Build history of the part. All positions in model axes, mm. Coordinates: 2 decimals unless noted, no trailing zeros. Loops run counter-clockwise (first coordinate to the right, second up) from the corner with the lowest first, then second, coordinate; pieces in that order, holes last. Notation, with made-up numbers: (-19, 19.5) -> (26, 19.5) arc R17 cw to (26, 42.5) -> close; hole circle Ø3 at (39.25, 50). An arc over 180 degrees is marked (long way). One line per item, written item: value. Start each with the question number.
Autodesk Inventor part; units mm, degrees
ref_plane "YZ Plane" through (0, 0, 0) normal (1, 0, 0) x (0, 1, 0)
ref_plane "XZ Plane" through (0, 0, 0) normal (0, 1, 0) x (-1, 0, 0)
ref_plane "XY Plane" through (0, 0, 0) normal (0, 0, 1) x (1, 0, 0)
sketch "Sketch1" plane through (0, 0, 0) normal (0, 1, 0) x (-1, 0, 0)
  line L0 (0, 0) -> (127, 0)
  line L1 (127, 0) -> (127, -127)
  line L2 (127, -127) -> (0, -127)
  line L3 (0, -127) -> (0, 0)
  line L4 (123.825, 0) -> (127, 0)
  line L5 (127, 0) -> (127, -33.615)
  line L6 (127, -33.615) -> (123.825, -33.615)
  line L7 (123.825, -33.615) -> (123.825, 0)
  line L8 (123.825, -33.615) -> (70.363, -33.615)
  line L9 (70.363, -33.615) -> (70.363, -36.79)
  line L10 (70.363, -36.79) -> (127, -36.79)
  line L11 (70.363, -36.79) -> (67.188, -36.79)
  line L12 (67.188, -36.79) -> (67.188, 0)
  line L13 (67.188, 0) -> (70.363, 0)
  line L14 (70.363, 0) -> (70.363, -36.79)
  line L15 (69.1283, -45.3517) -> (43.7283, -45.3517)
  line L16 (43.7283, -45.3517) -> (43.7283, -42.1767)
  line L17 (43.7283, -42.1767) -> (69.1283, -42.1767)
  line L18 (69.1283, -42.1767) -> (69.1283, -45.3517)
  line L19 (69.1283, -42.1767) -> (72.3033, -42.1767)
  line L20 (72.3033, -42.1767) -> (72.3033, -84.8107)
  line L21 (72.3033, -84.8107) -> (69.1283, -84.8107)
  line L22 (69.1283, -84.8107) -> (69.1283, -42.1767)
  line L23 (69.1283, -84.8107) -> (12.4863, -84.8107)
  line L24 (12.4863, -84.8107) -> (12.4863, -81.6357)
  line L25 (12.4863, -81.6357) -> (69.1283, -81.6357)
  line L26 (69.1283, -81.6357) -> (69.1283, -84.8107)
  line L27 (12.4863, -81.6357) -> (15.6613, -81.6357)
  line L28 (15.6613, -81.6357) -> (15.6613, -42.1767)
  line L29 (15.6613, -42.1767) -> (12.4863, -42.1767)
  line L30 (12.4863, -42.1767) -> (12.4863, -81.6357)
  line L31 (127, -90.21) -> (67.188, -90.21)
  line L32 (67.188, -90.21) -> (67.188, -93.385)
  line L33 (67.188, -93.385) -> (127, -93.385)
  line L34 (127, -93.385) -> (127, -90.21)
  line L35 (127, -93.385) -> (123.825, -93.385)
  line L36 (123.825, -93.385) -> (123.825, -127)
  line L37 (123.825, -127) -> (127, -127)
  line L38 (127, -127) -> (127, -93.385)
  line L39 (25.4, 0) -> (6.35, 0)
  line L40 (25.4, -127) -> (6.35, -127)
  line L41 (67.188, -90.21) -> (70.363, -90.21)
  line L42 (70.363, -90.21) -> (70.363, -127)
  line L43 (70.363, -127) -> (67.188, -127)
  line L44 (67.188, -127) -> (67.188, -90.21)
  line L45 (67.188, -3.175) -> (70.363, -3.175)
  line L46 (70.363, -3.175) -> (70.363, -33.615)
  line L47 (70.363, -33.615) -> (67.188, -33.615)
  line L48 (67.188, -33.615) -> (67.188, -3.175)
  line L49 (73.538, -33.615) -> (123.825, -33.615)
  line L50 (123.825, -33.615) -> (123.825, -36.79)
  line L51 (123.825, -36.79) -> (73.538, -36.79)
  line L52 (127, -3.175) -> (123.825, -3.175)
  line L53 (123.825, -3.175) -> (123.825, -30.44)
  line L54 (123.825, -30.44) -> (127, -30.44)
  line L55 (127, -30.44) -> (127, -3.175)
  line L56 (123.825, -90.21) -> (81.7068, -90.21)
  line L57 (81.7068, -93.385) -> (123.825, -93.385)
  line L58 (123.825, -93.385) -> (123.825, -90.21)
  line L59 (123.825, -96.56) -> (127, -96.56)
  line L60 (127, -96.56) -> (127, -123.825)
  line L61 (127, -123.825) -> (123.825, -123.825)
  line L62 (123.825, -123.825) -> (123.825, -96.56)
  line L63 (70.363, -96.56) -> (67.188, -96.56)
  line L64 (67.188, -96.56) -> (67.188, -123.825)
  line L65 (67.188, -123.825) -> (70.363, -123.825)
  line L66 (70.363, -123.825) -> (70.363, -96.56)
  line L67 (70.363, -30.44) -> (67.188, -30.44)
  line L68 (72.3033, -45.3517) -> (69.1283, -45.3517)
  line L69 (69.1283, -45.3517) -> (69.1283, -81.6357)
  line L70 (69.1283, -81.6357) -> (72.3033, -81.6357)
  line L71 (72.3033, -81.6357) -> (72.3033, -45.3517)
  line L72 (65.9533, -42.1767) -> (46.9033, -42.1767)
  line L73 (46.9033, -42.1767) -> (46.9033, -45.3517)
  line L74 (46.9033, -45.3517) -> (65.9533, -45.3517)
  line L75 (65.9533, -45.3517) -> (65.9533, -42.1767)
  line L76 (60.0198, -81.6357) -> (15.6613, -81.6357)
  line L77 (15.6613, -81.6357) -> (15.6613, -84.8107)
  line L78 (15.6613, -84.8107) -> (60.0198, -84.8107)
  line L79 (15.6613, -45.3517) -> (12.4863, -45.3517)
  line L80 (12.4863, -45.3517) -> (12.4863, -78.4607)
  line L81 (12.4863, -78.4607) -> (15.6613, -78.4607)
  line L82 (15.6613, -78.4607) -> (15.6613, -45.3517)
  line L83 (72.3033, -78.4607) -> (69.1283, -78.4607)
  line L84 (22.225, 0) -> (9.525, 0)
  line L85 (9.525, -127) -> (22.225, -127)
  line L86 (57.15, -3.175) -> (6.35, -3.175)
  line L87 (6.35, -3.175) -> (6.35, -6.35)
  line L88 (6.35, -6.35) -> (57.15, -6.35)
  line L89 (57.15, -6.35) -> (57.15, -3.175)
  line L90 (53.975, -3.175) -> (9.525, -3.175)
  line L91 (9.525, -3.175) -> (9.525, -6.35)
  line L92 (9.525, -6.35) -> (53.975, -6.35)
  line L93 (53.975, -6.35) -> (53.975, -3.175)
  line L94 (127, 0) -> (130.175, 0)
  line L95 (130.175, 0) -> (130.175, -127)
  line L96 (130.175, -127) -> (127, -127)
  line L97 (127, -127) -> (127, 0)
  line L98 (3.175, 0) -> (0, 0)
  line L99 (0, 0) -> (0, -127)
  line L100 (0, -127) -> (3.175, -127)
  line L101 (3.175, -127) -> (3.175, 0)
  line L102 (57.15, -120.65) -> (6.35, -120.65)
  line L103 (6.35, -120.65) -> (6.35, -123.825)
  line L104 (6.35, -123.825) -> (57.15, -123.825)
  line L105 (57.15, -123.825) -> (57.15, -120.65)
  line L106 (53.975, -120.65) -> (9.525, -120.65)
  line L107 (9.525, -120.65) -> (9.525, -123.825)
  line L108 (9.525, -123.825) -> (53.975, -123.825)
  line L109 (53.975, -123.825) -> (53.975, -120.65)
  line L110 (42.3948, -31.3817) -> (16.9948, -31.3817)
  line L111 (16.9948, -31.3817) -> (16.9948, -41.5417)
  line L112 (16.9948, -41.5417) -> (42.3948, -41.5417)
  line L113 (42.3948, -41.5417) -> (42.3948, -31.3817)
  line L114 (35.306, -9.525) -> (28.956, -9.525)
  line L115 (28.956, -9.525) -> (28.956, -12.7)
  line L116 (28.956, -12.7) -> (35.306, -12.7)
  line L117 (35.306, -12.7) -> (35.306, -9.525)
  line L118 (35.306, -25.0317) -> (28.956, -25.0317)
  line L119 (28.956, -25.0317) -> (28.956, -28.2067)
  line L120 (28.956, -28.2067) -> (35.306, -28.2067)
  line L121 (35.306, -28.2067) -> (35.306, -25.0317)
  line L122 (35.306, -44.7167) -> (28.956, -44.7167)
  line L123 (28.956, -44.7167) -> (28.956, -47.8917)
  line L124 (28.956, -47.8917) -> (35.306, -47.8917)
  line L125 (35.306, -47.8917) -> (35.306, -44.7167)
  line L126 (35.306, -87.9857) -> (28.956, -87.9857)
  line L127 (28.956, -87.9857) -> (28.956, -91.1607)
  line L128 (28.956, -91.1607) -> (35.306, -91.1607)
  line L129 (35.306, -91.1607) -> (35.306, -87.9857)
  line L130 (35.306, -114.3) -> (28.956, -114.3)
  line L131 (28.956, -114.3) -> (28.956, -117.475)
  line L132 (28.956, -117.475) -> (35.306, -117.475)
  line L133 (35.306, -117.475) -> (35.306, -114.3)
  point P0 (97.094, -33.615)
  point P1 (123.825, -110.1925)
  point P2 (123.825, -16.8075)
  point P3 (43.7283, -43.7642)
  point P4 (56.4283, -42.1767)
  point P5 (125.4125, 0)
  point P6 (125.4125, -3.175)
  point P7 (125.4125, -33.615)
  point P8 (70.363, -35.2025)
  point P9 (68.7755, -36.79)
  point P10 (68.7755, -33.615)
  point P11 (68.7755, 0)
  point P12 (68.7755, -3.175)
  point P13 (68.7755, -127)
  point P14 (68.7755, -123.825)
  point P15 (69.1283, -43.7642)
  point P16 (46.9033, -43.7642)
  point P17 (70.7158, -42.1767)
  point P18 (12.4863, -83.2232)
  point P19 (14.0738, -81.6357)
  point P20 (14.0738, -78.4607)
  point P21 (14.0738, -42.1767)
  point P22 (14.0738, -45.3517)
  point P23 (70.363, -93.385)
  point P24 (70.363, -30.44)
  point P25 (127, -96.56)
  point P26 (127, -30.44)
  point P27 (123.825, -33.615)
  point P28 (46.9033, -42.1767)
  point P29 (67.188, -96.56)
  point P30 (53.975, -4.7625)
  point P31 (53.975, -122.2375)
  point P32 (6.35, -122.2375)
  point P33 (15.875, -127)
  point P34 (127, -93.385)
  point P35 (53.975, -6.35)
  point P36 (32.131, -91.1607)
  dimension "d0" = 127
  dimension "d2" = 127
  dimension "d5" = 33.615
  dimension "d6" = 33.615
  dimension "d7" = 53.462
  dimension "d8" = 53.462
  dimension "d9" = 3.175
  dimension "d10" = 3.175
  dimension "d11" = 3.175
  dimension "d12" = 3.175
  dimension "d13" = 3.175
  dimension "d14" = 3.175
  dimension "d19" = 36.284
  dimension "d20" = 25.4
  dimension "d21" = 3.175
  dimension "d22" = 3.175
  dimension "d23" = 3.175
  dimension "d24" = 3.175
  dimension "d25" = 53.467
  dimension "d27" = 42.1767
  dimension "d28" = 3.175
  dimension "d29" = 3.175
  dimension "d30" = 3.175
  dimension "d32" = 3.175
  dimension "d33" = 3.175
  dimension "d34" = 3.175
  dimension "d35" = 3.175
  dimension "d36" = 3.175
  dimension "d37" = 3.175
  dimension "d38" = 3.175
  dimension "d39" = 3.175
  dimension "d40" = 3.175
  dimension "d41" = 3.175
  dimension "d42" = 3.175
  dimension "d43" = 3.175
  dimension "d44" = 3.175
  dimension "d45" = 3.175
  dimension "d46" = 3.175
  dimension "d51" = 3.175
  dimension "d52" = 3.175
  dimension "d53" = 3.175
  dimension "d54" = 50.8
  dimension "d55" = 3.175
  dimension "d56" = 6.35
  dimension "d57" = 3.175
  dimension "d58" = 3.175
  dimension "d59" = 3.175
  dimension "d60" = 3.175
  dimension "d61" = 3.175
  dimension "d62" = 50.8
  dimension "d63" = 6.35
  dimension "d64" = 3.175
  dimension "d65" = 9.3112
  dimension "d66" = 25.4
  dimension "d67" = 10.16
  dimension "d68" = 3.81
  dimension "d69" = 1.3335
  dimension "d70" = 6.35
  dimension "d71" = 3.175
  dimension "d72" = 3.175
  dimension "d73" = 6.35
  dimension "d74" = 3.175
  dimension "d75" = 3.175
  dimension "d76" = 6.35
extrude "Extrusion1" add sketch "Sketch1" along normal blind 3.175 contours L0 L12 L11 L10 L1 L31 L32 L44 L2 L101 | L0 L14 L45 L12 | L0 L7 L8 L14 | L44 L65 L42 L2 | L0 L1 L52 L7 | L67 L14 L47 L12 | L42 L33 L36 L2 | L94 L95 L96 L1 | L47 L9 L11 L12 | L36 L61 L1 L2 | L44 L33 L42 L63 | L54 L1 L6 L7 | L32 L31 L42 L33 | L6 L1 L10 L50 | L36 L33 L1 L59 | L58 L31 L1 L33 | L15 L75 L17 L18 | L18 L19 L20 L68 | L83 L20 L70 L22 | L15 L16 L17 L73 | L70 L20 L21 L22 | L77 L23 L24 L25 | L25 L30 L81 L28 | L79 L30 L29 L28 | L89 L88 L93 L86 | L91 L88 L87 L86 | L105 L104 L109 L102 | L107 L104 L103 L102
equation "\"d3\" = d41"
properties part number "top"
Item 1: Two-plate mould, pull along Z, no slides. Class faces 1 (the face through (-32, 2, -47.892)), 2 (the face through (-66, 2, 0)): +Z half, -Z half, draft (parallel to the pull), parting line (faces both ways), or undercut.
Item 2: Band-saw the part on C-C, the plane y = 1.85. Count the separate pieces of the cut face and the enclosed holes in it, and give its area (3 significant figures).
Item 3: Band-saw the part on A-A, the plane z = -103. List the corners of the cut face in (x, y) (3 decimals).
Item 4: Probe probe 1 along X at (y, z) = (1.85, -14) (3 decimals); probe 2 along X at (y, z) = (0.65, -10.5) (3 decimals); probe 3 along X at (y, z) = (1.65, -63) (3 decimals). List the from-to ranges inside material, lowest first.
Item 5: Band-saw the part on B-B, the plane x = -80.5. List the corners of the cut face in (y, z) (3 decimals), and give its area (3 significant figures).
Worked out:
1. face 1: undercut
1. face 2: +Z half
2. separate pieces: 1
2. enclosed holes: 18
2. area: 14,400 mm²
3. outline: (-130.175, 0) -> (-127, 0) -> (-127, 3.175) -> (-130.175, 3.175) -> close; (-123.825, 0) -> (-70.363, 0) -> (-70.363, 3.175) -> (-123.825, 3.175) -> close; (-67.188, 0) -> (-3.175, 0) -> (-3.175, 3.175) -> (-67.188, 3.175) -> close
4. probe 1: x = -130.175 to -127, -123.825 to -70.363, -67.188 to -3.175
4. probe 2: x = -130.175 to -127, -123.825 to -70.363, -67.188 to -35.306, -28.956 to -3.175
4. probe 3: x = -130.175 to -72.303, -69.128 to -15.661, -12.486 to -3.175
5. outline: (0, -127) -> (3.175, -127) -> (3.175, -93.385) -> (0, -93.385) -> close; (0, -90.21) -> (3.175, -90.21) -> (3.175, -36.79) -> (0, -36.79) -> close; (0, -33.615) -> (3.175, -33.615) -> (3.175, 0) -> (0, 0) -> close
5. area: 383 mm²
